Check sheet for the modelled part. Datum: model origin and axes. Units: mm. Coordinates: 2 decimals unless noted, no trailing zeros. Loops run counter-clockwise (first coordinate to the right, second up) from the corner with the lowest first, then second, coordinate; pieces in that order, holes last. Notation, with made-up numbers: M 23.25,81.5 L 64.25,81.5 A4 ccw 64.25,85.5 Z; hole C 26.25,58.25 d5. An arc over 180 degrees is marked long. Write each question's results on one line, items separated by ' | '. Start each with the question number.
from build123d import *
from OCP.BRepAlgoAPI import BRepAlgoAPI_Cut
from OCP.TopTools import TopTools_ListOfShape

# Parameters (mm, degrees)
SKETCH1_R           = 10.31875
SKETCH1_R_2         = 7.9375
BOSS_EXTRUDE1_DEPTH = 11.1125
CUT_EXTRUDE1_DEPTH  = 11.1125


with BuildPart() as part:
    # Sketch1 → Boss-Extrude1 (new body)
    with BuildSketch(Plane(origin=(0, 0, 0), x_dir=(1, 0, 0), z_dir=(0, 1, 0))):
        with Locations(Location((0, 0, 0), (0, 0, 270))):
            Circle(SKETCH1_R)
        with Locations(Location((0, 0, 0), (0, 0, 270))):
            Circle(SKETCH1_R_2, mode=Mode.SUBTRACT)
    extrude(amount=BOSS_EXTRUDE1_DEPTH)


with BuildPart() as cut_extrude1_tool:
    # Sketch2 → Cut-Extrude1 (new body)
    with BuildSketch(Plane(origin=(0, 11.1125, 0), x_dir=(1, 0, 0), z_dir=(0, 1, 0))):
        with BuildLine():
            ThreePointArc((0, 7.937497068), (1.378331901, 7.816908652), (2.714783885, 7.458807423))
            ThreePointArc((2.714783885, 7.458807423), (2.29060596, 7.757179042), (2.074464842, 8.228597701))
            ThreePointArc((2.074464842, 8.228597701), (1.473588959, 8.357138271), (0.864986861, 8.441861301))
            ThreePointArc((0.864986861, 8.441861301), (0.50064597, 8.072797282), (0, 7.937497068))
        make_face()
        with BuildLine():
            ThreePointArc((-2.714783885, 7.458807423), (-1.378331901, 7.816908652), (0, 7.937497068))
            ThreePointArc((0, 7.937497068), (-0.50064597, 8.072797282), (-0.864986861, 8.441861301))
            ThreePointArc((-0.864986861, 8.441861301), (-1.473588959, 8.357138271), (-2.074464842, 8.228597701))
            ThreePointArc((-2.074464842, 8.228597701), (-2.29060596, 7.757179042), (-2.714783885, 7.458807423))
        make_face()
        with BuildLine():
            ThreePointArc((-5.102124767, 6.080475521), (-3.968748534, 6.874074104), (-2.714783885, 7.458807423))
            ThreePointArc((-2.714783885, 7.458807423), (-3.231512607, 7.414717029), (-3.700108383, 7.636911841))
            ThreePointArc((-3.700108383, 7.636911841), (-4.2430303, 7.349144057), (-4.763705469, 7.022843776))
            ThreePointArc((-4.763705469, 7.022843776), (-4.805577005, 6.505930525), (-5.102124767, 6.080475521))
        make_face()
        with BuildLine():
            ThreePointArc((-6.874074104, 3.968748534), (-6.080475521, 5.102124767), (-5.102124767, 6.080475521))
            ThreePointArc((-5.102124767, 6.080475521), (-5.572611132, 5.862312472), (-6.088942225, 5.910838103))
            ThreePointArc((-6.088942225, 5.910838103), (-6.500699566, 5.454734609), (-6.878372912, 4.970031246))
            ThreePointArc((-6.878372912, 4.970031246), (-6.740924541, 4.469970769), (-6.874074104, 3.968748534))
        make_face()
        with BuildLine():
            ThreePointArc((-7.816908652, 1.378331901), (-7.458807423, 2.714783885), (-6.874074104, 3.968748534))
            ThreePointArc((-6.874074104, 3.968748534), (-7.241570511, 3.602826513), (-7.743359773, 3.471830055))
            ThreePointArc((-7.743359773, 3.471830055), (-7.974288525, 2.902403663), (-8.163407067, 2.317759598))
            ThreePointArc((-8.163407067, 2.317759598), (-7.863217092, 1.89486657), (-7.816908652, 1.378331901))
        make_face()
        with BuildLine():
            ThreePointArc((-7.816908652, -1.378331901), (-7.937497068, 0), (-7.816908652, 1.378331901))
            ThreePointArc((-7.816908652, 1.378331901), (-8.037089612, 0.908786504), (-8.463813852, 0.614068064))
            ThreePointArc((-8.463813852, 0.614068064), (-8.4860606, 0), (-8.463813852, -0.614068064))
            ThreePointArc((-8.463813852, -0.614068064), (-8.037089612, -0.908786504), (-7.816908652, -1.378331901))
        make_face()
        with BuildLine():
            ThreePointArc((-7.743359773, -3.471830055), (-7.241570511, -3.602826513), (-6.874074104, -3.968748534))
            ThreePointArc((-6.874074104, -3.968748534), (-7.458807423, -2.714783885), (-7.816908652, -1.378331901))
            ThreePointArc((-7.816908652, -1.378331901), (-7.863217092, -1.89486657), (-8.163407067, -2.317759598))
            ThreePointArc((-8.163407067, -2.317759598), (-7.974288525, -2.902403663), (-7.743359773, -3.471830055))
        make_face()
        with BuildLine():
            ThreePointArc((-6.088942225, -5.910838103), (-5.572611132, -5.862312472), (-5.102124767, -6.080475521))
            ThreePointArc((-5.102124767, -6.080475521), (-6.080475521, -5.102124767), (-6.874074104, -3.968748534))
            ThreePointArc((-6.874074104, -3.968748534), (-6.740924541, -4.469970769), (-6.878372912, -4.970031246))
            ThreePointArc((-6.878372912, -4.970031246), (-6.500699566, -5.454734609), (-6.088942225, -5.910838103))
        make_face()
        with BuildLine():
            ThreePointArc((-3.700108383, -7.636911841), (-3.231512607, -7.414717029), (-2.714783885, -7.458807423))
            ThreePointArc((-2.714783885, -7.458807423), (-3.968748534, -6.874074104), (-5.102124767, -6.080475521))
            ThreePointArc((-5.102124767, -6.080475521), (-4.805577005, -6.505930525), (-4.763705469, -7.022843776))
            ThreePointArc((-4.763705469, -7.022843776), (-4.2430303, -7.349144057), (-3.700108383, -7.636911841))
        make_face()
        with BuildLine():
            ThreePointArc((-0.864986861, -8.441861301), (-0.50064597, -8.072797282), (0, -7.937497068))
            ThreePointArc((0, -7.937497068), (-1.378331901, -7.816908652), (-2.714783885, -7.458807423))
            ThreePointArc((-2.714783885, -7.458807423), (-2.29060596, -7.757179042), (-2.074464842, -8.228597701))
            ThreePointArc((-2.074464842, -8.228597701), (-1.473588959, -8.357138271), (-0.864986861, -8.441861301))
        make_face()
        with BuildLine():
            ThreePointArc((2.074464842, -8.228597701), (2.29060596, -7.757179042), (2.714783885, -7.458807423))
            ThreePointArc((2.714783885, -7.458807423), (1.378331901, -7.816908652), (0, -7.937497068))
            ThreePointArc((0, -7.937497068), (0.50064597, -8.072797282), (0.864986861, -8.441861301))
            ThreePointArc((0.864986861, -8.441861301), (1.473588959, -8.357138271), (2.074464842, -8.228597701))
        make_face()
        with BuildLine():
            ThreePointArc((4.763705469, -7.022843776), (4.805577005, -6.505930525), (5.102124767, -6.080475521))
            ThreePointArc((5.102124767, -6.080475521), (3.968748534, -6.874074104), (2.714783885, -7.458807423))
            ThreePointArc((2.714783885, -7.458807423), (3.231512607, -7.414717029), (3.700108383, -7.636911841))
            ThreePointArc((3.700108383, -7.636911841), (4.2430303, -7.349144057), (4.763705469, -7.022843776))
        make_face()
        with BuildLine():
            ThreePointArc((6.878372912, -4.970031246), (6.740924541, -4.469970769), (6.874074104, -3.968748534))
            ThreePointArc((6.874074104, -3.968748534), (6.080475521, -5.102124767), (5.102124767, -6.080475521))
            ThreePointArc((5.102124767, -6.080475521), (5.572611132, -5.862312472), (6.088942225, -5.910838103))
            ThreePointArc((6.088942225, -5.910838103), (6.500699566, -5.454734609), (6.878372912, -4.970031246))
        make_face()
        with BuildLine():
            ThreePointArc((8.163407067, -2.317759598), (7.863217092, -1.89486657), (7.816908652, -1.378331901))
            ThreePointArc((7.816908652, -1.378331901), (7.458807423, -2.714783885), (6.874074104, -3.968748534))
            ThreePointArc((6.874074104, -3.968748534), (7.241570511, -3.602826513), (7.743359773, -3.471830055))
            ThreePointArc((7.743359773, -3.471830055), (7.974288525, -2.902403663), (8.163407067, -2.317759598))
        make_face()
        with BuildLine():
            ThreePointArc((5.102124767, 6.080475521), (6.080475521, 5.102124767), (6.874074104, 3.968748534))
            ThreePointArc((6.874074104, 3.968748534), (6.740924541, 4.469970769), (6.878372912, 4.970031246))
            ThreePointArc((6.878372912, 4.970031246), (6.500699566, 5.454734609), (6.088942225, 5.910838103))
            ThreePointArc((6.088942225, 5.910838103), (5.572611132, 5.862312472), (5.102124767, 6.080475521))
        make_face()
        with BuildLine():
            ThreePointArc((2.714783885, 7.458807423), (3.968748534, 6.874074104), (5.102124767, 6.080475521))
            ThreePointArc((5.102124767, 6.080475521), (4.805577005, 6.505930525), (4.763705469, 7.022843776))
            ThreePointArc((4.763705469, 7.022843776), (4.2430303, 7.349144057), (3.700108383, 7.636911841))
            ThreePointArc((3.700108383, 7.636911841), (3.231512607, 7.414717029), (2.714783885, 7.458807423))
        make_face()
        with BuildLine():
            ThreePointArc((6.874074104, 3.968748534), (7.458807423, 2.714783885), (7.816908652, 1.378331901))
            ThreePointArc((7.816908652, 1.378331901), (7.863217092, 1.89486657), (8.163407067, 2.317759598))
            ThreePointArc((8.163407067, 2.317759598), (7.974288525, 2.902403663), (7.743359773, 3.471830055))
            ThreePointArc((7.743359773, 3.471830055), (7.241570511, 3.602826513), (6.874074104, 3.968748534))
        make_face()
        with BuildLine():
            ThreePointArc((7.816908652, 1.378331901), (7.907292496, 0.691798453), (7.937497068, 0))
            ThreePointArc((7.937497068, 0), (7.907292496, -0.691798453), (7.816908652, -1.378331901))
            ThreePointArc((7.816908652, -1.378331901), (8.037089612, -0.908786504), (8.463813852, -0.614068064))
            ThreePointArc((8.463813852, -0.614068064), (8.480497089, -0.307235457), (8.4860606, 0))
            ThreePointArc((8.4860606, 0), (8.480497089, 0.307235457), (8.463813852, 0.614068064))
            ThreePointArc((8.463813852, 0.614068064), (8.037089612, 0.908786504), (7.816908652, 1.378331901))
        make_face()
    extrude(amount=-CUT_EXTRUDE1_DEPTH)


with BuildPart() as part_1:
    add(part.part)

    # Cut-Extrude1: cut by cut_extrude1_tool, with a tolerance
    cut_extrude1_stock = TopTools_ListOfShape()
    cut_extrude1_stock.Append(part_1.part.wrapped)
    cut_extrude1_tools = TopTools_ListOfShape()
    cut_extrude1_tools.Append(cut_extrude1_tool.part.wrapped)
    cut_extrude1_cut = BRepAlgoAPI_Cut()
    cut_extrude1_cut.SetArguments(cut_extrude1_stock)
    cut_extrude1_cut.SetTools(cut_extrude1_tools)
    cut_extrude1_cut.SetFuzzyValue(0.00001)
    cut_extrude1_cut.Build()
    add(Compound.cast(cut_extrude1_cut.Shape()).solids(), mode=Mode.REPLACE)


solid = part_1.part
1) Thickness scan on probe 1 along X at (y, z) = (3.25, -7.5); probe 2 along X at (y, z) = (9.25, 7.75); probe 3 along Z at (x, y) = (6, 5.5). Record the ranges inside material, lowest first.
2) Section check A-A (x = 1.75). Enter the section's corners in (y, z).
3) Gauge pin test, flat ends, axial feed: P1, Ø1, axis at x = 3, z = 5.5, coming from the +Y side; P2, Ø5, axis at y = 2.5, z = -8, coming from the -X side; P3, Ø5, axis at y = 8.5, z = 5, coming from the +X side; P4, Ø1.5, axis at x = -7, y = 8, coming from the -Z side. Record the tip position at first contact, or that the pin passes through.
4) Release check for a two-part mould opening along Z. For faces 1 (the cylindrical face through (10.23, 5.48, -1.34)), 2 (the cylindrical face through (-8.486, 5.634, -0.009)), 3 (the flat face through (5.4, 0, 6.1)) record: +Z half, -Z half, draft (parallel to the pull), parting line (faces both ways), or undercut.
Return value:
1) probe 1: x = -7.09 to -3.97, -3.49 to -2.62, 2.62 to 3.49, 3.97 to 7.09 | probe 2: x = -6.81 to -2.3, 2.3 to 6.81 | probe 3: z = -8.4 to -5.88, 5.88 to 8.4
2) outline: M 0,-10.17 L 11.11,-10.17 L 11.11,-8.3 L 0,-8.3 Z; M 0,8.3 L 11.11,8.3 L 11.11,10.17 L 0,10.17 Z
3) P1: passes through | P2: stops at x = -8.73 | P3: stops at x = 10.01 | P4: stops at z = -8.21
4) face 1: parting line | face 2: undercut | face 3: draft
